Part print with two shaded views. Sizes in mm from the minimum x, y, z corner. Give positions to 0.01 mm unless a question says otherwise; leave off trailing zeros. Order: outer loops, then holes, each group sorted by start corner. A loop starts at its lowest first (then second) coordinate and runs counter-clockwise, first axis right, second up. Notation, with made-up numbers: (25, 59.5) -> (82, 59.5) arc R7 cw to (82, 71.5) -> close; hole circle Ø5 at (-6.5, 7.25). An arc over 180 degrees is marked (long way). Write item = value, one per line. Start each with the question number.
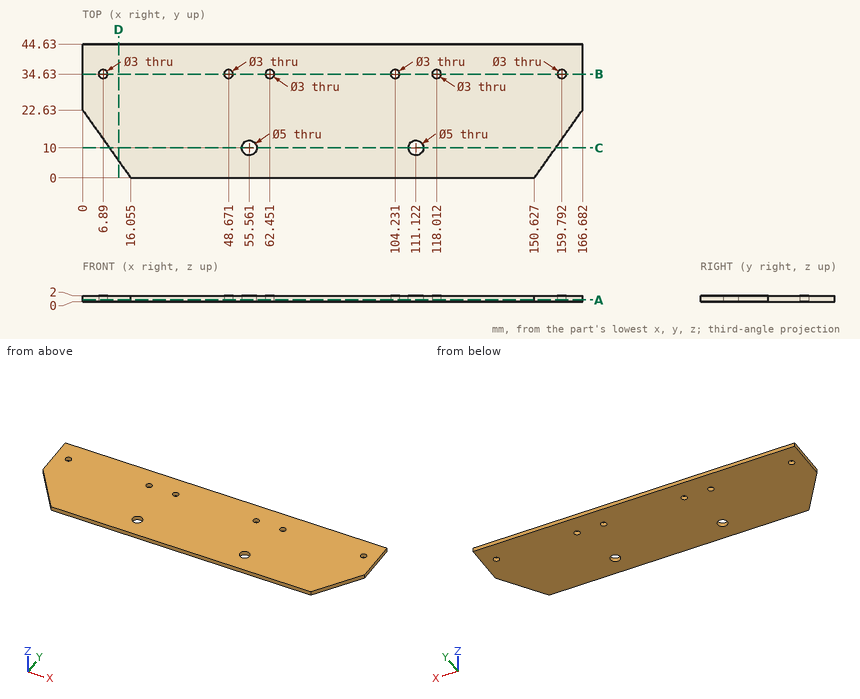
(1) Wall check: line 1 (X direction, y = 9, z = 1.4); line 2 (Y direction, x = 55.5, z = 1.4); line 3 (X direction, y = 8, z = 1.1) (1 decimal). Give the ranges that are in metal, low to high. Write a range as [from, to].
(2) Cut at D-D, the plane x = 12. Give the cut face in (y, z).
(3) Cut at A-A, the plane z = 0.7. Give the number of separate pieces and of enclosed holes in the cut face, plus the area to 3 significant figures.
(4) Cut at B-B, the plane y = 34.63. Give the cut face in (x, z).
(5) Cut at C-C, the plane y = 10. Give the cut face in (x, z).
(6) Flat gauge pin, fed straight in: P1, Ø6, axis at x = 55.56, y = 10, coming from the -Z side. Where does the tip first touch, or does it go through?
Results:
q1.line_1 = [9.67, 53.27], [57.85, 108.83], [113.41, 157.01]
q1.line_2 = [0, 7.5], [12.5, 44.63]
q1.line_3 = [10.4, 54.1], [57.1, 109.6], [112.6, 156.3]
q2.outline = (5.72, 0) -> (44.63, 0) -> (44.63, 2) -> (5.72, 2) -> close
q3.separate_pieces = 1
q3.enclosed_holes = 8
q3.area = 6,990 mm2
q4.outline = (0, 0) -> (5.39, 0) -> (5.39, 2) -> (0, 2) -> close; (8.39, 0) -> (47.17, 0) -> (47.17, 2) -> (8.39, 2) -> close; (50.17, 0) -> (60.95, 0) -> (60.95, 2) -> (50.17, 2) -> close; (63.95, 0) -> (102.73, 0) -> (102.73, 2) -> (63.95, 2) -> close; (105.73, 0) -> (116.51, 0) -> (116.51, 2) -> (105.73, 2) -> close; (119.51, 0) -> (158.29, 0) -> (158.29, 2) -> (119.51, 2) -> close; (161.29, 0) -> (166.68, 0) -> (166.68, 2) -> (161.29, 2) -> close
q5.outline = (8.96, 0) -> (53.06, 0) -> (53.06, 2) -> (8.96, 2) -> close; (58.06, 0) -> (108.62, 0) -> (108.62, 2) -> (58.06, 2) -> close; (113.62, 0) -> (157.72, 0) -> (157.72, 2) -> (113.62, 2) -> close
q6.P1 = 0
